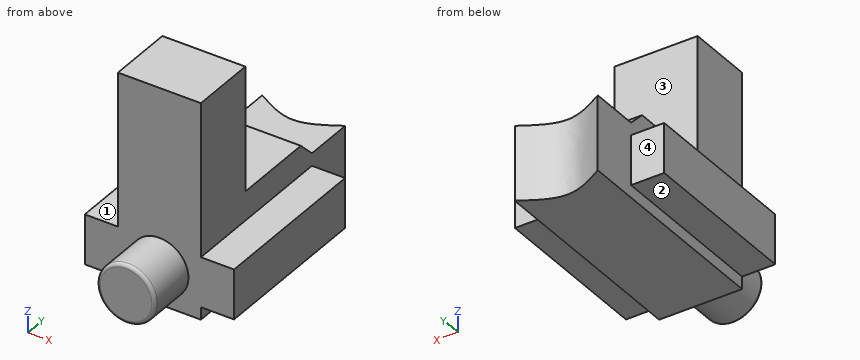
from build123d import *

# Parameters (mm, degrees)
F0_W     = 5
F0_H     = 7.5
F0_R     = 1.75
F0_H_2   = 1
F1_DEPTH = 4
F2_DEPTH = 3
F0_W_2   = 2
F0_H_3   = 3
F3_DEPTH = 10
F4_DEPTH = 13
F5_SIZE  = 0.99999
F7_DEPTH = 4.501
F8_R     = 0.2


# Not quite as in the source:
# - a fillet or chamfer is up to 0.001 mm smaller than in the source, because OpenCascade refuses the exact size


with BuildPart() as f1:
    # F0 (on Front) → F1 (new body)
    with BuildSketch(Plane.XZ):
        with Locations((2.5, 9.25)):
            Rectangle(F0_W, F0_H)
        Polygon((0, 0.75), (0, 0), (5, 0), (5, 0.75), (5, 3.75), (5, 4.5), (0, 4.5), (0, 3.75), align=None)
        with Locations((2.5, 2.25)):
            Circle(F0_R, mode=Mode.SUBTRACT)
        with Locations((2.5, 2.25)):
            Circle(F0_R)
        with Locations((2.5, 5)):
            Rectangle(F0_W, F0_H_2)
    extrude(amount=-F1_DEPTH)

    # F0 (on Front) → F2 (join)
    with BuildSketch(Plane.XZ):
        with Locations((2.5, 2.25)):
            Circle(F0_R)
    extrude(amount=F2_DEPTH)

    # F0 (on Front) → F3 (join)
    with BuildSketch(Plane.XZ):
        with Locations((6, 2.25)):
            Rectangle(F0_W_2, F0_H_3)
        with Locations((-1, 2.25)):
            Rectangle(F0_W_2, F0_H_3)
        with Locations((2.5, 5)):
            Rectangle(F0_W, F0_H_2)
        Polygon((0, 0.75), (0, 0), (5, 0), (5, 0.75), (5, 3.75), (5, 4.5), (0, 4.5), (0, 3.75), align=None)
        with Locations((2.5, 2.25)):
            Circle(F0_R, mode=Mode.SUBTRACT)
        with Locations((2.5, 2.25)):
            Circle(F0_R)
    extrude(amount=-F3_DEPTH)

    # F0 (on Front) → F4 (join)
    with BuildSketch(Plane.XZ):
        Polygon((0, 0.75), (0, 0), (5, 0), (5, 0.75), (5, 3.75), (5, 4.5), (0, 4.5), (0, 3.75), align=None)
        with Locations((2.5, 2.25)):
            Circle(F0_R, mode=Mode.SUBTRACT)
        with Locations((2.5, 2.25)):
            Circle(F0_R)
    extrude(amount=-F4_DEPTH)

    # F5 (size 1 in the source; OpenCascade refuses exactly that, so slightly less here)
    f5_edges = [f1.edges().sort_by_distance(p)[0] for p in [
        (2.5, 10, 5.5),
    ]]
    chamfer(f5_edges, length=F5_SIZE)

    # F6 (on face) → F7 (cut, through all)
    with BuildSketch(Plane.XY.offset(4.5)):
        with BuildLine():
            Line((5, 13), (2.5, 13))
            Line((2.5, 13), (2.5, 12))
            add(Edge.make_bspline(
                [(5, 13), (4.1666666667, 12.5), (3.3333333333, 12), (2.5, 12)],
                knots=[0, 0, 0, 0, 0.5, 0.5, 0.5, 0.5], degree=3))
        make_face()
        with BuildLine():
            Line((2.5, 12), (2.5, 13))
            Line((2.5, 13), (0, 13))
            add(Edge.make_bspline(
                [(2.5, 12), (1.6666666667, 12), (0.8333333333, 12.5), (0, 13)],
                knots=[0.5, 0.5, 0.5, 0.5, 1, 1, 1, 1], degree=3))
        make_face()
    extrude(amount=-F7_DEPTH, mode=Mode.SUBTRACT)

    # F8
    f8_edges = [f1.edges().sort_by_distance(p)[0] for p in [
        (0.75, -3, 2.25),
    ]]
    fillet(f8_edges, radius=F8_R)


solid = f1.part
Build history of the part. All positions in model axes, mm. Face numbers are marked on the shaded views. A direction names the side the tool comes from. Coordinates: 2 decimals unless noted, no trailing zeros. Order: outer loops, then holes, each group sorted by start corner. A loop starts at its lowest first (then second) coordinate and runs counter-clockwise, first axis right, second up. Notation, with made-up numbers: (13, -32) - (37, -32) arc R6 ccw to (37, -21) - close; hole circle Ø11 at (-15.5, 1.25). An arc over 180 degrees is marked (long way). Write each question's results on one line, items separated by ' | '. Start each with the question number.
Item 1: Band-saw the part on C-C on y = 1. Write the cut outline in (x, z), and give its area (3 significant figures).
Item 2: Band-saw the part on B-B on z = 10.75. Write the cut outline in (x, y), and give its area (3 significant figures).
Item 3: Band-saw the part on A-A on y = 4.25. Write the cut outline in (x, z).
Item 4: Tool access for the marked faces 1, 2, 3 and 4: list every direction of +Z, -Z, +X, -X, +Y, -Y with a clear straight run to the whole face (end or side of a thin tool).
Item 5: Wall check: probe 1 along Z at (x, y) = (2.5, 8); probe 2 along Y at (x, z) = (4.5, 6.25); probe 3 along Z at (x, y) = (6.5, 4). Give the ranges that are in metal, low to high. Write a range as [from, to].
Item 6: Flat gauge pins, fed straight in: pin 1 (4 mm diameter, centred on y = 2, z = 5, fed in from -X); pin 2 (1.6 mm diameter, centred on x = 6, z = 2.5, fed in from +Y); pin 3 (1.6 mm diameter, centred on x = 6, y = 5.5, fed in from +Z); pin 4 (2.5 mm diameter, centred on x = 3, y = 6.5, fed in from +Z). Where does each tip first touch, or does it go through?
Numbers:
1) outline: (-2, 0.75) - (0, 0.75) - (0, 0) - (5, 0) - (5, 0.75) - (7, 0.75) - (7, 3.75) - (5, 3.75) - (5, 13) - (0, 13) - (0, 3.75) - (-2, 3.75) - close | area: 77.0 mm^2
2) outline: (0, 0) - (5, 0) - (5, 4) - (0, 4) - close | area: 20.0 mm^2
3) outline: (-2, 0.75) - (0, 0.75) - (0, 0) - (5, 0) - (5, 0.75) - (7, 0.75) - (7, 3.75) - (5, 3.75) - (5, 5.5) - (0, 5.5) - (0, 3.75) - (-2, 3.75) - close
4) face 1: +Z, -X, +Y, -Y | face 2: -Z, -X, +Y, -Y | face 3: +Z, +X, -X, +Y | face 4: +Z, -Z, -X, +Y
5) probe 1: [0, 5.5] | probe 2: [0, 4] | probe 3: [0.75, 3.75]
6) pin 1: x = -2 | pin 2: y = 10 | pin 3: z = 3.75 | pin 4: z = 5.5
